Answer from the drawing. Dimensions are ordinates in mm from the lowest x, y and z of the part. Coordinates: 2 decimals unless noted, no trailing zeros. Loops run counter-clockwise (first coordinate to the right, second up) from the corner with the lowest first, then second, coordinate; pieces in that order, holes last.
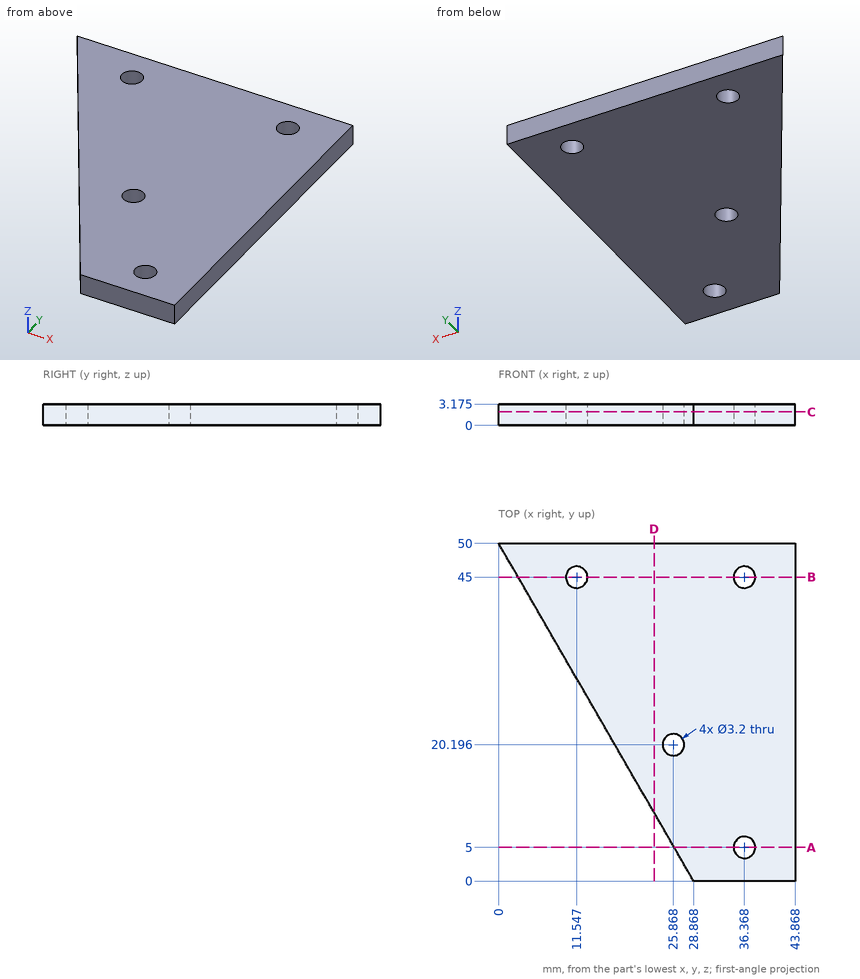
Item 1: A cutting plane is placed at D-D on x = 23. Determine the outline of the cut face in (y, z) (1 decimal).
Numbers:
outline: (10.2, 0) - (50, 0) - (50, 3.2) - (10.2, 3.2) - close
Item 2: Find the intervals of material crossed by line 1 along X through (y, z) = (45.5, 0.7) (1 decimal); line 2 along Y through (x, z) = (10.5, 1.05) (1 decimal); line 3 along X through (y, z) = (4, 0.95) (1 decimal), in increasing order.
Numbers:
line 1: x = 2.6 to 10, 13.1 to 34.8, 37.9 to 43.9
line 2: y = 31.8 to 43.8, 46.2 to 50
line 3: x = 26.6 to 35.1, 37.6 to 43.9
Item 3: A cutting plane is placed at A-A on y = 5. Determine the outline of the cut face in (x, z) (1 decimal).
Numbers:
outline: (26, 0) - (34.8, 0) - (34.8, 3.2) - (26, 3.2) - close; (38, 0) - (43.9, 0) - (43.9, 3.2) - (38, 3.2) - close
Item 4: A cutting plane is placed at B-B on y = 45. Determine the outline of the cut face in (x, z) (1 decimal), then the cut area to 3 significant figures.
Numbers:
outline: (2.9, 0) - (9.9, 0) - (9.9, 3.2) - (2.9, 3.2) - close; (13.1, 0) - (34.8, 0) - (34.8, 3.2) - (13.1, 3.2) - close; (38, 0) - (43.9, 0) - (43.9, 3.2) - (38, 3.2) - close
area: 110 mm2
Item 5: Given pin 1 (8 mm diameter, centred on x = 15.5, y = 26, fed in from -Z); pin 2 (1.5 mm diameter, centred on y = 19, z = 0.5, fed in from -X) (1 decimal), each flat-ended and moving along its own axis, determine where each tip first touches the part or whether it passes through.
Numbers:
pin 1: stops at z = 0
pin 2: stops at x = 17.5
Item 6: A cutting plane is placed at C-C on z = 2. Determine the outline of the cut face in (x, y).
Numbers:
outline: (0, 50) - (28.87, 0) - (43.87, 0) - (43.87, 50) - close; hole circle Ø3.2 at (11.55, 45); hole circle Ø3.2 at (25.87, 20.2); hole circle Ø3.2 at (36.37, 5); hole circle Ø3.2 at (36.37, 45)
